Part model, mm, in its own coordinate system. A direction names the side the tool comes from. Coordinates: 2 decimals unless noted, no trailing zeros. Loops run counter-clockwise (first coordinate to the right, second up) from the corner with the lowest first, then second, coordinate; pieces in that order, holes last. Notation, with made-up numbers: (88.25, 47) - (124.25, 47) arc R13 ccw to (124.25, 67) - close; hole circle Ø9 at (-4, 63). An arc over 180 degrees is marked (long way). One line per question, with ' | ' between items. Start each with the question number.
from build123d import *

# Parameters (mm, degrees)
SKETCH2_W           = 160
SKETCH2_H           = 88.569233124
BOSS_EXTRUDE1_DEPTH = 10
SKETCH3_W           = 10
SKETCH3_H           = 88.569233124
BOSS_EXTRUDE2_DEPTH = 152.4
SKETCH4_W           = 10
SKETCH4_H           = 5
CUT_EXTRUDE6_DEPTH  = 152.4
SKETCH4_2_W         = 10
SKETCH4_2_H         = 5
BOSS_EXTRUDE3_DEPTH = 5
SKETCH6_W           = 10
SKETCH6_H           = 88.569233124
BOSS_EXTRUDE4_DEPTH = 5


with BuildPart() as part:
    # Sketch2 → Boss-Extrude1 (new body)
    with BuildSketch(Plane(origin=(0, 0, 0), x_dir=(0, 0, -1), z_dir=(1, 0, 0))):
        Rectangle(SKETCH2_W, SKETCH2_H)
    boss_extrude1 = extrude(amount=BOSS_EXTRUDE1_DEPTH)

    # Sketch3 → Boss-Extrude2 (add)
    with BuildSketch(Plane.ZY):
        with Locations((-75, 0)):
            Rectangle(SKETCH3_W, SKETCH3_H)
    extrude(amount=BOSS_EXTRUDE2_DEPTH)

    # Sketch4 → Cut-Extrude6 (cut)
    with BuildSketch(Plane.ZY.offset(152.4)):
        with Locations((-75, 0)):
            Rectangle(SKETCH4_W, SKETCH4_H)
    extrude(amount=-CUT_EXTRUDE6_DEPTH, mode=Mode.SUBTRACT)

    # Sketch4<2> → Boss-Extrude3 (add)
    with BuildSketch(Plane.ZY.offset(152.4)):
        with Locations((-75, 0)):
            Rectangle(SKETCH4_2_W, SKETCH4_2_H)
    extrude(amount=-BOSS_EXTRUDE3_DEPTH)

    # Sketch6 → Boss-Extrude4 (add)
    with BuildSketch(Plane(origin=(10, 0, 0), x_dir=(0, 0, -1), z_dir=(1, 0, 0))):
        with Locations((32.47, 0)):
            Rectangle(SKETCH6_W, SKETCH6_H)
        with Locations((-47.53, 0)):
            Rectangle(SKETCH6_W, SKETCH6_H)
    boss_extrude4 = extrude(amount=BOSS_EXTRUDE4_DEPTH)

    # Mirror2: Boss-Extrude1, Boss-Extrude4 across plane
    add(boss_extrude1.mirror(Plane(origin=(0, 0, 0), x_dir=(0, 0, 1), z_dir=(1, 0, 0))))
    add(boss_extrude4.mirror(Plane(origin=(0, 0, 0), x_dir=(0, 0, 1), z_dir=(1, 0, 0))))


solid = part.part
1) Pin check, flat tips, straight feed: pin 1 Ø2.5 at (y, z) = (-1, -76) entering from +X; pin 2 Ø1 at (y, z) = (3.5, 55.5) entering from -X; pin 3 Ø1.5 at (y, z) = (19.5, 52) entering from -X. Stop position of each tip, or through.
2) Band-saw the part on B-B on y = 38. List the corners of the cut face in (x, z), then the cut area to 3 significant figures.
3) Band-saw the part on D-D on z = 47. List the corners of the cut face in (x, y), then the cut area to 3 significant figures.
4) Mould opens along Z. For faces 1 (the flat face through (-10, 1, 8)), 2 (the flat face through (12, -1, -37.47)), 3 (the flat face through (-152.4, 1, -75)) say: +Z half, -Z half, draft (parallel to the pull), parting line (faces both ways), or undercut.
5) Wall check: line 1 along X through (y, z) = (34.5, 71); line 2 along Z through (x, y) = (-67.5, -26.5); line 3 along X through (y, z) = (-14, 43.5). Give the ranges that are in metal, low to high. Write a range as [from, to].
6) Band-saw the part on C-C on z = 1. List the corners of the cut face in (x, y).
7) Band-saw the part on A-A on x = -61. List the corners of the cut face in (y, z).
8) Tool access for faces 4 (the flat face through (12, -1, 42.53)), 5 (the flat face through (-10, 1, 66)), 6 (the flat face through (-12, -1, -27.47)), 7 (the flat face through (10, 1, 66)): list every direction of +Z, -Z, +X, -X, +Y, -Y with a clear straight run to the whole face (end or side of a thin tool).
Values found:
1) pin 1: x = 10 | pin 2: x = -10 | pin 3: x = -15
2) outline: (-152.4, -80) - (10, -80) - (10, -37.47) - (15, -37.47) - (15, -27.47) - (10, -27.47) - (10, 42.53) - (15, 42.53) - (15, 52.53) - (10, 52.53) - (10, 80) - (-10, 80) - (-10, 52.53) - (-15, 52.53) - (-15, 42.53) - (-10, 42.53) - (-10, -27.47) - (-15, -27.47) - (-15, -37.47) - (-10, -37.47) - (-10, -70) - (-152.4, -70) - close | area: 4,820 mm²
3) outline: (-15, -44.28) - (15, -44.28) - (15, 44.28) - (-15, 44.28) - close | area: 2,660 mm²
4) face 1: undercut | face 2: -Z half | face 3: draft
5) line 1: [-10, 10] | line 2: [-80, -70] | line 3: [-15, 15]
6) outline: (-10, -44.28) - (10, -44.28) - (10, 44.28) - (-10, 44.28) - close
7) outline: (-44.28, -80) - (-2.5, -80) - (-2.5, -70) - (-44.28, -70) - close; (2.5, -80) - (44.28, -80) - (44.28, -70) - (2.5, -70) - close
8) face 4: +X, +Y, -Y | face 5: +Z, -X, +Y, -Y | face 6: -X, +Y, -Y | face 7: +Z, +X, +Y, -Y
